Source: CAD feature listing. Evaluate the final solid. Frame: model axes, mm. A direction names the side the tool comes from. Give positions to 0.01 mm unless a question says otherwise; leave off trailing zeros. Loops run counter-clockwise (first coordinate to the right, second up) from the corner with the lowest first, then second, coordinate; pieces in that order, holes last. Notation, with made-up numbers: (80.5, 73) -> (104.5, 73) arc R16 cw to (104.5, 95) -> close; hole circle Ø3 at (24, 5). An arc over 180 degrees is marked (long way). Return JSON: item names as keys, results as strings. Group by question number.
(1) Pin query (flat end, axial travel): pin 1 (5 mm diameter, centred on y = -13.5, z = 10, fed in from -X); pin 2 (5.5 mm diameter, centred on x = 14.5, z = 6.5, fed in from +Y); pin 3 (7 mm diameter, centred on y = -4.5, z = 7.5, fed in from +X); pin 4 (3 mm diameter, centred on x = 16, z = 7.05, fed in from +Y). Return the tip coordinate at first contact, or that it passes through.
(2) Draft query along Y for faces 1 (the face through (-5, 13.42, 7)), 2 (the face through (20.96, -17, 7)), 3 (the face through (4.984, 9.946, 7.531)). Return one class per face: released by +Y, released by -Y, zero draft, split by the parting line, or undercut.
(3) Ray query, line 1 (Z direction, x = -7.3, y = 8.42); line 2 (X direction, y = 7, z = 3.5); line 3 (X direction, y = 0, z = 5.75). Return the intervals inside material, ascending. Write a range as from..to.
(4) Cut plane D-D on y = -16.5. Return loops of the section in (x, z), then the cut area to 3 significant figures.
(5) Cut plane C-C on x = 7. Return loops of the section in (y, z), then the cut area to 3 significant figures.
(6) Cut plane B-B on y = 8.42. Return loops of the section in (x, z) (3 decimals).
(7) Cut plane A-A on x = 16. Return loops of the section in (y, z).
(8) Access query for faces 4 (the face through (-2.956, 6.393, 7.688)), 5 (the face through (-0.7, 11, 7)), 6 (the face through (9.15, 0, 7)). Directions: +Z, -Z, +X, -X, +Y, -Y. A direction counts if a zero-diameter tool reaches every point of the face in a straight line with its end or side. Return the directions, or none.
```python
from build123d import *

# Parameters (mm, degrees)
F1_DEPTH = 14.1
F2_R     = 1.6
F3_DEPTH = 30.111
F4_R     = 4
F5_DEPTH = 4
F6_R     = 2.66
F7_DEPTH = 25
F8_R     = 2.125
F9_DEPTH = 5.85
F10_R    = 0.5
F11_SIZE = 0.25


with BuildPart() as f1:
    # F0 (on Top) → F1 (new body)
    with BuildSketch(Plane.XY):
        with BuildLine():
            ThreePointArc((0.7, 4.9507575178), (0, -5), (-0.7, 4.9507575178))
            Line((-0.7, 4.9507575178), (-0.7, 13.42))
            Line((-0.7, 13.42), (-9.15, 13.42))
            Line((-9.15, 13.42), (-9.15, -13.12))
            Line((-9.15, -13.12), (-20.96, -13.12))
            Line((-20.96, -13.12), (-20.96, -20))
            Line((-20.96, -20), (20.96, -20))
            Line((20.96, -20), (20.96, -13.12))
            Line((20.96, -13.12), (9.15, -13.12))
            Line((9.15, -13.12), (9.15, 13.42))
            Line((9.15, 13.42), (0.7, 13.42))
            Line((0.7, 13.42), (0.7, 4.9507575178))
        make_face()
    extrude(amount=F1_DEPTH)

    # F2 (on face) → F3 (cut, through all)
    with BuildSketch(Plane.YZ.offset(9.15)):
        with Locations((8.42, 7.05)):
            Circle(F2_R)
    extrude(amount=-F3_DEPTH, mode=Mode.SUBTRACT)

    # F4 (on face) → F5 (cut)
    with BuildSketch(Plane(origin=(-9.15, 0, 0), x_dir=(0, -1, 0), z_dir=(-1, 0, 0))):
        with Locations((-8.42, 7.05)):
            Circle(F4_R)
    extrude(amount=-F5_DEPTH, mode=Mode.SUBTRACT)

    # F6 (on face) → F7 (cut)
    with BuildSketch(Plane.XZ.offset(20)):
        with Locations((-16, 7.05)):
            Circle(F6_R)
        with Locations((16, 7.05)):
            Circle(F6_R)
    extrude(amount=-F7_DEPTH, mode=Mode.SUBTRACT)

    # F8 (on face) → F9 (cut, through all)
    with BuildSketch(Plane(origin=(-5.15, 0, 0), x_dir=(0, -1, 0), z_dir=(-1, 0, 0))):
        with Locations((-8.42, 7.05)):
            Circle(F8_R)
    extrude(amount=-F9_DEPTH, mode=Mode.SUBTRACT)

    # F10
    f10_edges = [f1.edges().sort_by_distance(p)[0] for p in [
        (-20.96, -13.12, 7.05),
        (-20.96, -20, 7.05),
        (20.96, -13.12, 7.05),
        (20.96, -20, 7.05),
        (9.15, 13.42, 7.05),
        (-9.15, 13.42, 7.05),
        (0, -5, 14.1),
        (0, -5, 0),
    ]]
    fillet(f10_edges, radius=F10_R)

    # F11
    f11_edges = [f1.edges().sort_by_distance(p)[0] for p in [
        (13.34, -20, 7.05),
        (18.66, -16.56, 7.05),
        (13.34, -13.12, 7.05),
        (-18.66, -20, 7.05),
        (-13.34, -16.56, 7.05),
        (-18.66, -13.12, 7.05),
    ]]
    chamfer(f11_edges, length=F11_SIZE)


solid = f1.part
```
Answers:
{
 "1": {"pin 1": "x = -20.96", "pin 2": "y = -13.12", "pin 3": "x = 9.15", "pin 4": "through"},
 "2": {"face 1": "released by +Y", "face 2": "zero draft", "face 3": "undercut"},
 "3": {"line 1": "0..3.05, 11.05..14.1", "line 2": "-5.15..-0.7, 0.7..9.15", "line 3": "-9.15..-5, 5..9.15"},
 "4": {"outline": "(-20.96, 0) -> (20.96, 0) -> (20.96, 14.1) -> (-20.96, 14.1) -> close; hole circle Ø5.32 at (-16, 7.05); hole circle Ø5.32 at (16, 7.05)", "area": "547 mm²"},
 "5": {"outline": "(-20, 0) -> (13.42, 0) -> (13.42, 14.1) -> (-20, 14.1) -> close; hole circle Ø3.2 at (8.42, 7.05)", "area": "463 mm²"},
 "6": {"outline": "(-9.15, 0) -> (-0.7, 0) -> (-0.7, 4.925) -> (-5.15, 4.925) -> (-5.15, 3.05) -> (-9.15, 3.05) -> close; (-9.15, 11.05) -> (-5.15, 11.05) -> (-5.15, 9.175) -> (-0.7, 9.175) -> (-0.7, 14.1) -> (-9.15, 14.1) -> close; (0.7, 0) -> (9.15, 0) -> (9.15, 5.45) -> (0.7, 5.45) -> close; (0.7, 8.65) -> (9.15, 8.65) -> (9.15, 14.1) -> (0.7, 14.1) -> close"},
 "7": {"outline": "(-20, 0) -> (-13.12, 0) -> (-13.12, 4.14) -> (-13.37, 4.39) -> (-19.75, 4.39) -> (-20, 4.14) -> close; (-20, 9.96) -> (-19.75, 9.71) -> (-13.37, 9.71) -> (-13.12, 9.96) -> (-13.12, 14.1) -> (-20, 14.1) -> close"},
 "8": {"face 4": "-X", "face 5": "+Z, -Z, +Y", "face 6": "+Z, -Z, +X, +Y"}
}
